Autodesk Inventor part; units mm, degrees
ref_plane "YZ Plane" through (0, 0, 0) normal (1, 0, 0) x (0, 1, 0)
ref_plane "XZ Plane" through (0, 0, 0) normal (0, 1, 0) x (-1, 0, 0)
ref_plane "XY Plane" through (0, 0, 0) normal (0, 0, 1) x (1, 0, 0)
sketch "スケッチ1" plane through (0, 0, 0) normal (0, 1, 0) x (-1, 0, 0)
  circle A0 centre (0, 0) radius 60
  line L0 (60, 0) -> (-60, 0)
  line L1 (-60, 0) -> (-60, 47)
  line L2 (-60, 47) -> (60, 47)
  line L3 (60, 47) -> (60, 0)
  line L4 (9.5, -70) -> (9.5, -59.2431)
  line L5 (-9.5, -70) -> (-9.5, -59.2431)
  line L6 (9.5, -70) -> (-9.5, -70)
  line L7 (0, -70) -> (0, -60)
  point P0 (37.2961, 47)
  point P1 (3.75, -60.165)
  point P2 (-3.75, -60.165)
  point P3 (-37.2961, 47)
  dimension "d41" = 120
  dimension "d70" = 60.165
  dimension "d71" = 7.5
  dimension "d72" = 3.75
  dimension "d88" = 47
  dimension "d147" = 19
  dimension "d148" = 10
extrude "押し出し1" add sketch "スケッチ1" along normal blind 1.6 contours L0 A0 | L1 L2 A0 | A0 L2 L0 | A0 L7 L6 L5 | A0 L2 L3 | A0 L4 L6 L7
sketch "スケッチ6" plane through (0, 1.6, 0) normal (0, 1, 0) x (-1, 0, 0)
  line L0 (-33.4, -30) -> (-33.4, 42) construction
  line L1 (-33.4, 42) -> (-38.4, 42) construction
  line L2 (-38.4, 42) -> (-38.4, -30) construction
  line L3 (-33.4, 12) -> (-38.4, 12) construction
  line L4 (-40.9, 21.5) -> (-40.9, -18.5) construction
  line L5 (-33.4, -30) -> (-38.4, -30) construction
  line L6 (-42.5, 20) -> (-42.5, -20) construction
  point P0 (0, 0)
  point P1 (-35.9, 0)
  dimension "d52" = 5
  dimension "d53" = 72
  dimension "d54" = 30
  dimension "d55" = 2.5
  dimension "d68" = 33.4
  dimension "d69" = 12
  dimension "d100" = 30
hole "穴3" at (33.4, 1.6, 42) at (38.4, 1.6, 42) at (38.4, 1.6, -30) at (33.4, 1.6, -30) at (35.9, 1.6, 0) direction (0, -1, 0) diameter 2.4 end through all
mirror "ミラー2" about plane through (0, 0, 0) normal (1, 0, 0) of "穴3"
sketch "スケッチ9" plane through (0, 1.6, 0) normal (0, 1, 0) x (1, 0, 0)
  line L0 (-40.9, 23) -> (-70.9, 23)
  line L1 (-70.9, 23) -> (-70.9, -32)
  line L2 (-70.9, -32) -> (-40.9, -32)
  line L3 (-40.9, -32) -> (-40.9, 23)
  line L4 (-60, 0) -> (-60, -47)
  line L5 (-60, -47) -> (60, -47)
  line L6 (-40.9, -32) -> (-70.9, -32)
  line L7 (-70.9, -32) -> (-70.9, -49)
  line L8 (-70.9, -49) -> (-40.9, -49)
  line L9 (-40.9, -49) -> (-40.9, -32)
  point P0 (0, 0)
  point P1 (-40.9, -47)
  point P2 (-60, -32)
  dimension "d84" = 55
  dimension "d89" = 23
  dimension "d90" = 40.9
  dimension "d91" = 30
  dimension "d92" = 17
extrude "押し出し2" cut sketch "スケッチ9" against normal blind 10 contours L3 L2 L1 L0 | L9 L5 L4 L2
mirror "ミラー3" about plane through (0, 0, 0) normal (1, 0, 0) of "押し出し2"
sketch "スケッチ12" plane through (0, 1.6, 0) normal (0, 1, 0) x (1, 0, 0)
  line L0 (-56.8017, 16.1133) -> (59.6732, 16.1133) construction
  line L1 (59.6732, 16.1133) -> (59.6732, -15.1509) construction
  line L2 (59.6732, -15.1509) -> (-56.8017, -15.1509) construction
  line L3 (-56.8017, -15.1509) -> (-56.8017, 16.1133) construction
  point P0 (0, 0)
sketch "スケッチ13" plane through (0, 1.6, 0) normal (0, 1, 0) x (1, 0, 0)
  point P0 (0, 0)
fillet "フィレット1" radius 10 2 edges at (9.5, 0.8, -59.2431) (-9.5, 0.8, -59.2431)
sketch "スケッチ16" plane through (0, 0, 0) normal (0, -1, 0) x (1, 0, 0)
  circle A0 centre (-35.9, 0) radius 1.2
  line L0 (-33.4, -7.5) -> (-38.4, -7.5)
  line L1 (-38.4, -7.5) -> (-38.4, 7.5)
  line L2 (-38.4, 7.5) -> (-33.4, 7.5)
  line L3 (-33.4, 7.5) -> (-33.4, -7.5)
  line L4 (-33.4, -7.5) -> (-38.4, 7.5) construction
  line L5 (-33.4, 7.5) -> (-38.4, -7.5) construction
  point P0 (0, 0)
  point P1 (-35.9, 0)
  dimension "d120" = 5
  dimension "d121" = 15
extrude "押し出し4" cut sketch "スケッチ16" against normal blind 10
fillet "フィレット2" radius 2 4 edges at (-33.4, 0.8, -7.5) (-33.4, 0.8, 7.5) (-38.4, 0.8, 7.5) (-38.4, 0.8, -7.5)
mirror "ミラー5" about plane through (0, 0, 0) normal (1, 0, 0) of "押し出し4", "フィレット2"
sketch "スケッチ21" plane through (0, 1.6, 0) normal (0, 1, 0) x (1, 0, 0)
  line L0 (9.5, 72.5) -> (-9.5, 72.5)
  line L1 (-9.5, 70) -> (9.5, 70)
  line L2 (9.5, 70) -> (9.5, 60)
  line L3 (9.5, 60) -> (-9.5, 60)
  line L4 (-9.5, 60) -> (-9.5, 70)
  line L5 (0, 70) -> (0, 67.5)
  line L6 (-3.1667, 67.5) -> (0, 67.5)
  line L7 (0, 62.5) -> (-3.1667, 62.5)
  line L8 (-3.1667, 62.5) -> (-3.1667, 67.5)
  circle A0 centre (-6.3333, 65) radius 1.5833
  line L9 (0, 65) -> (-1.5833, 65) construction
  line L10 (-1.5833, 65) -> (-3.1667, 65) construction
  line L11 (-3.1667, 65) -> (-4.75, 65) construction
  line L12 (-4.75, 65) -> (-6.3333, 65) construction
  line L13 (-6.3333, 65) -> (-7.9167, 65) construction
  line L14 (-7.9167, 65) -> (-9.5, 65) construction
  line L15 (3.1667, 67.5) -> (0, 67.5)
  line L16 (0, 62.5) -> (3.1667, 62.5)
  line L17 (3.1667, 62.5) -> (3.1667, 67.5)
  circle A1 centre (6.3333, 65) radius 1.5833
  line L18 (0, 65) -> (0, 62.5)
  line L19 (0, 67.5) -> (0, 65)
  line L20 (0, 62.5) -> (0, 60)
  point P0 (0, 0)
  dimension "d146" = 10
extrude "押し出し7" cut sketch "スケッチ21" against normal blind 1.6 contours L19 L18 L7 L8 L6 | L15 L17 L16 L18 L19
sketch "スケッチ22" plane through (0, 1.6, 0) normal (0, 1, 0) x (1, 0, 0)
  line L0 (-3.1667, 67.5) -> (-3.1667, 62.5)
  line L1 (-3.1667, 65) -> (-9.5, 65)
  line L2 (-9.5, 70) -> (-9.5, 67.2291)
  line L3 (-3.1667, 67.5) -> (3.1667, 67.5)
  line L4 (0, 67.5) -> (0, 65.9167)
  point P0 (0, 0)
  point P1 (-6.3333, 65)
  point P2 (6.3333, 65)
hole "穴8" at (-6.3333, 1.6, -65) at (6.3333, 1.6, -65) direction (0, -1, 0) diameter 2.4 end through all
fillet "フィレット5" radius 1.5 4 edges at (-3.1667, 0.8, -67.5) (-3.1667, 0.8, -62.5) (3.1667, 0.8, -62.5) (3.1667, 0.8, -67.5)
ref_plane "作業平面5" through (0, 0, -23) normal (1, 0, 0) x (0, 0, -1)
properties part number "flame" material "エポキシ樹脂"
Part model, mm, in its own coordinate system. Round coordinates to 2 decimals unless told otherwise and drop trailing zeros. Write each loop counter-clockwise with the first axis right and the second up, starting at its lowest first coordinate (ties: lowest second). Pieces come first, ordered by that corner, then holes. Notation, with made-up numbers: M 87,-23 L 100,-23 A11 ccw 100,-12 Z; hole C 88,-18 d11. An arc over 180 degrees is marked long. One line per question, with ' | ' between items.
(1) Saw through at C-C on y = 0.8. Count the separate pieces of the cut face and the enclosed holes in it, then the cut area to 3 significant figures.
Answer key:
separate pieces: 1 | enclosed holes: 13 | area: 8,690 mm^2
(2) Pin check, flat tips, straight feed: pin 1 (4 mm diameter, centred on x = -38.4, z = 42, fed in from +Y); pin 2 (0.8 mm diameter, centred on y = 0.5, z = 1, fed in from +X); pin 3 (0.5 mm diameter, centred on x = -51, y = 1, fed in from +Z); pin 4 (1.9 mm diameter, centred on x = -6.33, z = -65, fed in from +Y). Stop position of each tip, or through.
Answer key:
pin 1: stops at y = 1.6 | pin 2: stops at x = 40.9 | pin 3: stops at z = -23 | pin 4: passes through
(3) Saw through at A-A on z = 12. Write the cut outline in (x, y).
Answer key:
outline: M -40.9,0 L 40.9,0 L 40.9,1.6 L -40.9,1.6 Z
(4) Saw through at B-B on x = 23. Write the cut outline in (y, z), then the cut area to 3 significant figures.
Answer key:
outline: M 0,-55.42 L 1.6,-55.42 L 1.6,47 L 0,47 Z | area: 164 mm^2
(5) Probe line 1 along X through (y, z) = (1.15, -2.5); line 2 along X through (y, z) = (0.6, 42); line 3 along X through (y, z) = (0.5, -30). List the from-to ranges inside material, lowest first.
Answer key:
line 1: x = -40.9 to -38.4, -33.4 to 33.4, 38.4 to 40.9 | line 2: x = -40.9 to -39.6, -37.2 to -34.6, -32.2 to 32.2, 34.6 to 37.2, 39.6 to 40.9 | line 3: x = -51.96 to -39.6, -37.2 to -34.6, -32.2 to 32.2, 34.6 to 37.2, 39.6 to 51.96
